from build123d import *

# Parameters (mm, degrees)
BOSS_EXTRUDE1_DEPTH     = 21.7
SKETCH2_R               = 1.75
CUT_EXTRUDE1_DEPTH      = 10
SKETCH3_W               = 35.7
SKETCH3_H               = 71
BOSS_EXTRUDE2_DEPTH     = 35
SKETCH4_W               = 20.2
SKETCH4_H               = 20.2
CUT_EXTRUDE2_DEPTH      = 72
SKETCH5_R               = 2.75
CUT_EXTRUDE3_DEPTH      = 10
MIRROR5_COPY_1_SKETCH_R = 2.75
MIRROR5_COPY_1_DEPTH    = 10
MIRROR5_COPY_2_SKETCH_R = 2.75
MIRROR5_COPY_2_DEPTH    = 10
MIRROR6_COPY_1_SKETCH_R = 2.75
MIRROR6_COPY_1_DEPTH    = 10
FILLET1_R               = 3
FILLET2_R               = 1


with BuildPart() as part:
    # Sketch1 → Boss-Extrude1 (new body)
    with BuildSketch(Plane.XY):
        Polygon((27.75, 0), (-27.75, 0), (-27.75, 56), (-12.75, 56), (-12.75, 8), (12.75, 8), (12.75, 56), (27.75, 56), align=None)
    extrude(amount=BOSS_EXTRUDE1_DEPTH)

    # Sketch2 → Cut-Extrude1 (cut)
    with BuildSketch(Plane(origin=(0, 56, 0), x_dir=(1, 0, 0), z_dir=(0, 1, 0))):
        with Locations((20.25, -6)):
            Circle(SKETCH2_R)
        with Locations((20.25, -15.7)):
            Circle(SKETCH2_R)
        with Locations((-20.25, -15.7)):
            Circle(SKETCH2_R)
        with Locations((-20.25, -6)):
            Circle(SKETCH2_R)
    extrude(amount=-CUT_EXTRUDE1_DEPTH, mode=Mode.SUBTRACT)

    # Sketch3 → Boss-Extrude2 (add)
    with BuildSketch(Plane(origin=(27.75, 0, 0), x_dir=(0, 0, -1), z_dir=(1, 0, 0))):
        with Locations((-10.85, 35.5)):
            Rectangle(SKETCH3_W, SKETCH3_H)
    boss_extrude2 = extrude(amount=BOSS_EXTRUDE2_DEPTH)

    # Mirror1: Boss-Extrude2 across plane
    add(boss_extrude2.mirror(Plane(origin=(0, 0, 0), x_dir=(0, 0, 1), z_dir=(1, 0, 0))))

    # Sketch4 → Cut-Extrude2 (cut, through all)
    with BuildSketch(Plane.XZ):
        with Locations((45.25, 10.85)):
            Rectangle(SKETCH4_W, SKETCH4_H)
    cut_extrude2 = extrude(amount=-CUT_EXTRUDE2_DEPTH, mode=Mode.SUBTRACT)

    # Mirror2: Cut-Extrude2 across plane
    add(cut_extrude2.mirror(Plane(origin=(0, 0, 0), x_dir=(0, 0, 1), z_dir=(1, 0, 0))), mode=Mode.SUBTRACT)

    # Sketch5 → Cut-Extrude3 (cut)
    with BuildSketch(Plane.XY.offset(28.7)):
        with Locations((45.25, 51)):
            Circle(SKETCH5_R)
        with Locations((45.25, 20)):
            Circle(SKETCH5_R)
    cut_extrude3 = extrude(amount=-CUT_EXTRUDE3_DEPTH, mode=Mode.SUBTRACT)

    # Mirror3: Cut-Extrude3 across plane
    add(cut_extrude3.mirror(Plane(origin=(0, 0, 0), x_dir=(0, 0, 1), z_dir=(1, 0, 0))), mode=Mode.SUBTRACT)

    # Mirror4: Cut-Extrude3 across plane
    add(cut_extrude3.mirror(Plane(origin=(17.649039404, 0, -17.302979808), x_dir=(0.700071411, 0, 0.714072839), z_dir=(0.714072839, 0, -0.700071411))), mode=Mode.SUBTRACT)

    # Mirror5 copy 1 sketch → Mirror5 copy 1 (cut)
    with BuildSketch(Plane(origin=(-63.99245246, 0, -34.03769849), x_dir=(0.019800039, 0, 0.99980396), z_dir=(-0.99980396, 0, 0.019800039))):
        with Locations((45.25, 51)):
            Circle(MIRROR5_COPY_1_SKETCH_R)
        with Locations((45.25, 20)):
            Circle(MIRROR5_COPY_1_SKETCH_R)
    extrude(amount=-MIRROR5_COPY_1_DEPTH, mode=Mode.SUBTRACT)

    # Mirror5 copy 2 sketch → Mirror5 copy 2 (cut)
    with BuildSketch(Plane(origin=(-63.99245246, 0, -34.03769849), x_dir=(-0.019800039, 0, -0.99980396), z_dir=(-0.99980396, 0, 0.019800039))):
        with Locations((45.25, -51)):
            Circle(MIRROR5_COPY_2_SKETCH_R)
        with Locations((45.25, -20)):
            Circle(MIRROR5_COPY_2_SKETCH_R)
    extrude(amount=-MIRROR5_COPY_2_DEPTH, mode=Mode.SUBTRACT)

    # Mirror6: Cut-Extrude3 across plane
    add(cut_extrude3.mirror(Plane(origin=(0, 0, 10.85), x_dir=(1, 0, 0), z_dir=(0, 0, -1))), mode=Mode.SUBTRACT)

    # Mirror6 copy 1 sketch → Mirror6 copy 1 (cut)
    with BuildSketch(Plane(origin=(0, 0, -7), x_dir=(-1, 0, 0), z_dir=(0, 0, -1))):
        with Locations((45.25, 51)):
            Circle(MIRROR6_COPY_1_SKETCH_R)
        with Locations((45.25, 20)):
            Circle(MIRROR6_COPY_1_SKETCH_R)
    extrude(amount=-MIRROR6_COPY_1_DEPTH, mode=Mode.SUBTRACT)

    # Fillet1
    fillet1_edges = [part.edges().sort_by_distance(p)[0] for p in [
        (27.75, 35.5, -7),
        (27.75, 35.5, 28.7),
        (62.75, 35.5, -7),
        (62.75, 35.5, 28.7),
        (-27.75, 35.5, -7),
        (-27.75, 35.5, 28.7),
        (-62.75, 35.5, -7),
        (-62.75, 35.5, 28.7),
    ]]
    fillet(fillet1_edges, radius=FILLET1_R)

    # Fillet2
    fillet2_edges = [part.edges().sort_by_distance(p)[0] for p in [
        (-45.25, 71, 28.7),
        (-45.25, 0, 28.7),
        (45.25, 0, -7),
        (62.75, 0, 10.85),
        (45.25, 0, 28.7),
        (27.75, 0, 23.7),
        (-27.75, 0, 23.7),
        (-62.75, 0, 10.85),
        (-45.25, 0, -7),
        (-61.871320344, 0, -6.121320344),
        (-28.628679656, 0, -6.121320344),
        (28.628679656, 0, -6.121320344),
        (61.871320344, 0, -6.121320344),
        (61.871320344, 0, 27.821320344),
        (28.628679656, 0, 27.821320344),
        (-28.628679656, 0, 27.821320344),
        (-61.871320344, 0, 27.821320344),
        (-62.75, 71, 10.85),
        (-27.75, 71, 10.85),
        (-45.25, 71, -7),
        (-61.871320344, 71, -6.121320344),
        (-28.628679656, 71, -6.121320344),
        (-28.628679656, 71, 27.821320344),
        (-61.871320344, 71, 27.821320344),
        (45.25, 71, 28.7),
        (27.75, 71, 10.85),
        (62.75, 71, 10.85),
        (45.25, 71, -7),
        (28.628679656, 71, -6.121320344),
        (61.871320344, 71, -6.121320344),
        (61.871320344, 71, 27.821320344),
        (28.628679656, 71, 27.821320344),
        (0, 0, 21.7),
        (27.75, 0, -2),
        (-27.75, 0, -2),
        (0, 0, 0),
    ]]
    fillet(fillet2_edges, radius=FILLET2_R)


solid = part.part
Design review of the part built by this model. Coordinates are the model's own, in mm. A direction names the side the tool comes from. Coordinates: 2 decimals unless noted, no trailing zeros. Write each loop counter-clockwise with the first axis right and the second up, starting at its lowest first coordinate (ties: lowest second). Pieces come first, ordered by that corner, then holes. Notation, with made-up numbers: (-36, 80) - (-14, 80) arc R13 cw to (-14, 101) - close; hole circle Ø10 at (84, -34.5). An arc over 180 degrees is marked (long way). Use one line per item in the form item = value.
Q1. Machinability: for faces 5 (the cylindrical face through (28.61, 35.98, 27.8)), 6 (the flat face through (12.75, 32, 11)), 7 (the cylindrical face through (-21.64, 51.07, 7.06)), 8 (the flat face through (55.35, 35, 11)), which of the approach directions +Z, -Z, +X, -X, +Y, -Y give a long, thin tool a straight path to every point of the face, cutting with its end or side? Answer none if there is none.
Taken from the geometry:
face_5 = +Z, +Y, -Y
face_6 = +Z, -Z, +Y
face_7 = +Y
face_8 = +Y, -Y
Q2. For probe 1 along X at (y, z) = (38, 3); probe 2 along Y at (x, z) = (-45, -3); probe 3 along X at (y, z) = (49.5, 15.7), list the stretches that pass through material, from the lowest coordinate up.
Taken from the geometry:
probe_1 = -62.75 to -55.35, -35.15 to -12.75, 12.75 to 35.15, 55.35 to 62.75
probe_2 = 0 to 17.26, 22.74 to 48.26, 53.74 to 71
probe_3 = -62.75 to -55.35, -35.15 to -22, -18.5 to -12.75, 12.75 to 18.5, 22 to 35.15, 55.35 to 62.75
Q3. Consider section A-A (y = 44.5). Count the separate pieces of the cut face and the enclosed holes in it, plus the area to 3 significant figures.
Taken from the geometry:
separate_pieces = 2
enclosed_holes = 2
area = 2,320 mm^2
Q4. Consider section D-D (x = 8). Write out the cut boundary in (y, z), plus the area to 3 significant figures.
Taken from the geometry:
outline = (0, 1) arc R1 ccw to (1, 0) - (8, 0) - (8, 21.7) - (1, 21.7) arc R1 ccw to (0, 20.7) - close
area = 173 mm^2
Q5. The part is to be moulded in two halves that separate along Y. For faces 1 (the cylindrical face through (59.11, 22.727, 10.766)), 2 (the flat face through (20, 56, 11)), 3 (the flat face through (1, 0, 11)), 4 (the flat face through (-12.75, 32, 11)), say which applies: +Y half, -Y half, draft (parallel to the pull), parting line (faces both ways), or undercut.
Taken from the geometry:
face_1 = undercut
face_2 = +Y half
face_3 = -Y half
face_4 = draft
Q6. Insertion check: pin 1 Ø1.8 at (x, z) = (-20.5, 15.5) entering from +Y; pin 2 Ø1 at (x, z) = (9, 6.5) entering from +Y; pin 3 Ø16.5 at (x, y) = (5, 32.5) entering from +Z. Each pin has a flat end and moves straight along its axis. Give the tip position at first contact, or say it passes through.
Taken from the geometry:
pin_1 = 46
pin_2 = 8
pin_3 = 21.7
Q7. Consider section C-C (x = -45.25). Write out the cut boundary in (y, z).
Taken from the geometry:
outline = (0, -6) arc R1 ccw to (1, -7) - (17.25, -7) - (17.25, 0.75) - (0, 0.75) - close; (0, 20.95) - (17.25, 20.95) - (17.25, 28.7) - (1, 28.7) arc R1 ccw to (0, 27.7) - close; (22.75, -7) - (48.25, -7) - (48.25, 0.75) - (22.75, 0.75) - close; (22.75, 20.95) - (48.25, 20.95) - (48.25, 28.7) - (22.75, 28.7) - close; (53.75, -7) - (70, -7) arc R1 ccw to (71, -6) - (71, 0.75) - (53.75, 0.75) - close; (53.75, 20.95) - (71, 20.95) - (71, 27.7) arc R1 ccw to (70, 28.7) - (53.75, 28.7) - close
